CAD build for the part. Positions are in the model's coordinates, mm. A direction names the side the tool comes from. Give positions to 0.01 mm unless a question says otherwise; leave off trailing zeros. Write each loop counter-clockwise with the first axis right and the second up, starting at its lowest first coordinate (ties: lowest second). Pieces come first, ordered by that corner, then holes. Notation, with made-up numbers: (-28.5, 20.5) - (-0.5, 20.5) arc R20 cw to (-0.5, 30.5) - close; hole circle Ø10 at (-34.75, 59.25). An arc over 180 degrees is marked (long way). Put each result on its own line as item: value. Start each with the question number.
1. Mould opens along Y. For faces 5 (the cylindrical face through (6.725, -5.981, 0.774)), 6 (the flat face through (0, 2.45, 2)), 7 (the cylindrical face through (0.59, -6.93, 0.77)) say: +Y half, -Y half, draft (parallel to the pull), parting line (faces both ways), or undercut.
2. Drop flat-ended pins along their axis: pin 1 (1.4 mm diameter, centred on x = -0.5, z = 2.5, fed in from -Y); pin 2 (1 mm diameter, centred on x = -0.5, y = -4, fed in from +Z); pin 3 (0.5 mm diameter, centred on x = -1, z = 2.5, fed in from +Y). Give the stop position or say it passes through.
3. Wall check: line 1 (Y direction, x = 0, z = 0.95); line 2 (Z direction, x = 5, y = 6); line 3 (X direction, y = -2.25, z = 3.05). Give the ranges that are in metal, low to high.
4. Cut at A-A on x = 0. List the corners of the cut face in (y, z).
5. Tool access for faces 1 (the flat face through (-1.95, 0, 2)), 2 (the cylindrical face through (6.68, 6.03, 0.77)), 3 (the flat face through (1.95, 0, 2)), 4 (the flat face through (0, -2.45, 2)): list every direction of +Z, -Z, +X, -X, +Y, -Y with a clear straight run to the whole face (end or side of a thin tool).
6. Cut at D-D on y = 1.5. List the corners of the cut face in (x, z), and give its area (3 significant figures).
7. Cut at B-B on y = -6. List the corners of the cut face in (x, z), and give its area (3 significant figures).
8. Cut at C-C on z = 0.9. List the corners of the cut face in (x, y).
Autodesk Inventor part; units mm, degrees
ref_plane "YZ Plane" through (0, 0, 0) normal (1, 0, 0) x (0, 1, 0)
ref_plane "XZ Plane" through (0, 0, 0) normal (0, 1, 0) x (-1, 0, 0)
ref_plane "XY Plane" through (0, 0, 0) normal (0, 0, 1) x (1, 0, 0)
sketch "Sketch1" plane through (0, 0, 0) normal (0, 0, 1) x (1, 0, 0)
  line L0 (8, 7.5) -> (4.9749, 7.5) construction
  line L1 (-8, 7.5) -> (-8, 4.1231) construction
  line L2 (-8, -7.5) -> (-4.9749, -7.5) construction
  line L3 (8, -7.5) -> (8, -4.1231) construction
  arc A0 (8, 4.1231) -> (4.9749, 7.5) centre (0, 0) ccw
  arc A1 (8, -4.1231) -> (8, 4.1231) centre (0, 0) ccw construction
  arc A2 (-4.9749, 7.5) -> (-8, 4.1231) centre (0, 0) ccw
  arc A3 (-4.9749, -7.5) -> (4.9749, -7.5) centre (0, 0) ccw construction
  arc A4 (4.9749, -7.5) -> (8, -4.1231) centre (0, 0) ccw
  line L4 (4.9749, -7.5) -> (8, -7.5) construction
  line L5 (-4.9749, -7.5) -> (4.9749, -7.5)
  line L6 (-8, -4.1231) -> (-8, -7.5) construction
  line L7 (8, 4.1231) -> (8, 7.5) construction
  line L8 (8, -4.1231) -> (8, 4.1231)
  line L9 (-8, 4.1231) -> (-8, -4.1231)
  line L10 (-4.9749, 7.5) -> (-8, 7.5) construction
  arc A5 (4.9749, 7.5) -> (-4.9749, 7.5) centre (0, 0) ccw construction
  arc A6 (-8, 4.1231) -> (-8, -4.1231) centre (0, 0) ccw construction
  arc A7 (-8, -4.1231) -> (-4.9749, -7.5) centre (0, 0) ccw
  line L11 (4.9749, 7.5) -> (-4.9749, 7.5)
  circle A8 centre (0, -6) radius 1.1
  circle A9 centre (0, 6) radius 1.1
  dimension "d3" = 15
  dimension "d4" = 16
  dimension "d6" = 7.5
  dimension "d7" = 8
  dimension "d8" = 18
  dimension "d9" = 6
  dimension "d10" = 2.2
  dimension "d11" = 2.2
  dimension "d12" = 6
extrude "Extrusion1" add sketch "Sketch1" along normal blind 1.57
sketch "Sketch2" plane through (0, 0, 1.57) normal (0, 0, 1) x (1, 0, 0)
  line L0 (1.95, 2.45) -> (-1.95, 2.45)
  line L1 (-1.95, 2.45) -> (-1.95, -2.45)
  line L2 (-1.95, -2.45) -> (1.95, -2.45)
  line L3 (1.95, -2.45) -> (1.95, 2.45)
  point P0 (0, 0)
  dimension "d15" = 4.9
  dimension "d16" = 3.9
  dimension "d17" = 1.95
  dimension "d18" = 2.45
extrude "Extrusion2" add sketch "Sketch2" along normal blind 1.75
sketch "Sketch3" plane through (0, 0, 3.32) normal (0, 0, 1) x (1, 0, 0)
  circle A0 centre (0, 0) radius 1.4142
  dimension "d21" = 2.8284
properties part number "AS5600"
Report:
1. face 5: -Y half
1. face 6: +Y half
1. face 7: undercut
2. pin 1: stops at y = -2.45
2. pin 2: stops at z = 1.57
2. pin 3: stops at y = 2.45
3. line 1: y = -7.5 to -7.1, -4.9 to 4.9, 7.1 to 7.5
3. line 2: z = 0 to 1.57
3. line 3: x = -1.95 to 1.95
4. outline: (-7.5, 0) - (-7.1, 0) - (-7.1, 1.57) - (-7.5, 1.57) - close; (-4.9, 0) - (4.9, 0) - (4.9, 1.57) - (2.45, 1.57) - (2.45, 3.32) - (-2.45, 3.32) - (-2.45, 1.57) - (-4.9, 1.57) - close; (7.1, 0) - (7.5, 0) - (7.5, 1.57) - (7.1, 1.57) - close
5. face 1: +Z, -X, +Y, -Y
5. face 2: +Z, -Z, +X, +Y
5. face 3: +Z, +X, +Y, -Y
5. face 4: +Z, +X, -X, -Y
6. outline: (-8, 0) - (8, 0) - (8, 1.57) - (1.95, 1.57) - (1.95, 3.32) - (-1.95, 3.32) - (-1.95, 1.57) - (-8, 1.57) - close
6. area: 31.9 mm²
7. outline: (-6.71, 0) - (-1.1, 0) - (-1.1, 1.57) - (-6.71, 1.57) - close; (1.1, 0) - (6.71, 0) - (6.71, 1.57) - (1.1, 1.57) - close
7. area: 17.6 mm²
8. outline: (-8, -4.12) arc R9 ccw to (-4.97, -7.5) - (4.97, -7.5) arc R9 ccw to (8, -4.12) - (8, 4.12) arc R9 ccw to (4.97, 7.5) - (-4.97, 7.5) arc R9 ccw to (-8, 4.12) - close; hole circle Ø2.2 at (0, -6); hole circle Ø2.2 at (0, 6)
